The listing builds one solid part. Answer for the finished solid, in the listing's coordinates (mm). A direction names the side the tool comes from. Coordinates: 2 decimals unless noted, no trailing zeros. Write each loop counter-clockwise with the first axis right and the second up, starting at its lowest first coordinate (ties: lowest second). Pieces come first, ordered by that corner, then holes.
```python
from build123d import *

# Parameters (mm, degrees)
CROQUIS1_W              = 5.95
CROQUIS1_H              = 5.95
SALIENTE_EXTRUIR1_DEPTH = 3.5
CROQUIS3_R              = 1.7
SALIENTE_EXTRUIR2_DEPTH = 1.5
CROQUIS4_R              = 0.5
SALIENTE_EXTRUIR3_DEPTH = 0.4
CROQUIS5_W              = 1.355791782
CROQUIS5_H              = 0.82
SALIENTE_EXTRUIR4_DEPTH = 0.405
REDONDEO1_R             = 0.3
REDONDEO2_R             = 0.3
CROQUIS9_W              = 1.36
CROQUIS9_H              = 0.82
SALIENTE_EXTRUIR5_DEPTH = 0.405
REDONDEO3_R             = 0.3
REDONDEO4_R             = 0.3
CORTAR_EXTRUIR1_DEPTH   = 10.958472837


with BuildPart() as part:
    # Croquis1 → Saliente-Extruir1 (new body)
    with BuildSketch(Plane.XY):
        with Locations((-2.975, 2.975)):
            Rectangle(CROQUIS1_W, CROQUIS1_H)
    extrude(amount=SALIENTE_EXTRUIR1_DEPTH)

    # Croquis3 → Saliente-Extruir2 (add)
    with BuildSketch(Plane.XY.offset(3.5)):
        with Locations((-2.975, 2.975)):
            Circle(CROQUIS3_R)
    extrude(amount=SALIENTE_EXTRUIR2_DEPTH)

    # Croquis4 → Saliente-Extruir3 (add)
    with BuildSketch(Plane.XY.offset(3.5)):
        with Locations((-5.25, 5.3125)):
            Circle(CROQUIS4_R)
        with Locations(Location((-0.7, 5.3125, 0), (0, 0, 180))):
            Circle(CROQUIS4_R)
        with Locations((-0.7, 0.6375)):
            Circle(CROQUIS4_R)
        with Locations(Location((-5.25, 0.6375, 0), (0, 0, 180))):
            Circle(CROQUIS4_R)
    extrude(amount=SALIENTE_EXTRUIR3_DEPTH)

    # Croquis5 → Saliente-Extruir4 (add)
    with BuildSketch(Plane(origin=(0, 0, 0), x_dir=(0, 0, -1), z_dir=(1, 0, 0))):
        with Locations((-0.677895891, 5.4025)):
            Rectangle(CROQUIS5_W, CROQUIS5_H)
        with Locations((-0.677895891, 0.5475)):
            Rectangle(CROQUIS5_W, CROQUIS5_H)
    extrude(amount=SALIENTE_EXTRUIR4_DEPTH)

    # Redondeo1
    redondeo1_edges = [part.edges().sort_by_distance(p)[0] for p in [
        (0.405, 5.4025, 1.355791782),
    ]]
    fillet(redondeo1_edges, radius=REDONDEO1_R)

    # Redondeo2
    redondeo2_edges = [part.edges().sort_by_distance(p)[0] for p in [
        (0.405, 0.5475, 1.355791782),
    ]]
    fillet(redondeo2_edges, radius=REDONDEO2_R)

    # Croquis9 → Saliente-Extruir5 (add)
    with BuildSketch(Plane.ZY.offset(5.95)):
        with Locations((0.68, 5.4025)):
            Rectangle(CROQUIS9_W, CROQUIS9_H)
        with Locations((0.68, 0.5475)):
            Rectangle(CROQUIS9_W, CROQUIS9_H)
    extrude(amount=SALIENTE_EXTRUIR5_DEPTH)

    # Redondeo3
    redondeo3_edges = [part.edges().sort_by_distance(p)[0] for p in [
        (-6.355, 5.4025, 1.36),
    ]]
    fillet(redondeo3_edges, radius=REDONDEO3_R)

    # Redondeo4
    redondeo4_edges = [part.edges().sort_by_distance(p)[0] for p in [
        (-6.355, 0.5475, 1.36),
    ]]
    fillet(redondeo4_edges, radius=REDONDEO4_R)

    # Croquis10 → Cortar-Extruir1 (cut, through all)
    with BuildSketch(Plane.XZ.offset(-0.1375)):
        with BuildLine():
            Line((-5.95, 0), (-6.055, 0))
            Line((-6.055, 0), (-6.055, 0.955))
            ThreePointArc((-6.055, 0.955), (-6.024246212, 1.029246212), (-5.95, 1.06))
            Line((-5.95, 1.06), (-5.95, 0))
        make_face()
        with BuildLine():
            Line((0.105, 0), (0.105, 0.955))
            ThreePointArc((0.105, 0.955), (0.074246212, 1.029246212), (0, 1.06))
            Line((0, 1.06), (0, 0))
            Line((0, 0), (0.105, 0))
        make_face()
    extrude(amount=-CORTAR_EXTRUIR1_DEPTH, mode=Mode.SUBTRACT)


solid = part.part
```
(1) Section C-C, the plane y = 0.5 is taken. Write down the section's boundary in (x, z) (3 decimals), plus the area to 3 significant figures.
(2) Section D-D, the plane z = 2.35 is taken. Write down the section's boundary in (x, y).
(3) Which of the six approach directions +Z, -Z, +X, -X, +Y, -Y give full straight-line access (tool end or side, diameter ignored) to faces 1 (the flat face through (-4.34, 1.69, 3.5)), 2 (the flat face through (-0.7, 0.6, 3.9))?
(4) Each of these flat-tipped pins is pushed along its axis until it touches: pin 1 (1.8 mm diameter, centred on y = 2, z = 2, fed in from +X); pin 2 (1.1 mm diameter, centred on x = -0.5, y = 1, fed in from +Z). Where does it stop, or does it pass through?
(5) Section A-A, the plane z = 0.4 is taken. State how many separate pieces and enclosed holes the cut face has, plus the area to 3 significant figures.
(6) For a pull along X with two mould halves and no side action, classify faces 3 (the flat face through (0.405, 0.6, 0.5)), 4 (the flat face through (-0.7, 5.3, 3.9)), 5 (the cylindrical face through (-0.635, 4.817, 3.697)) as pulls with the +X half, pulls with the -X half, needs draft (parallel to the pull), parting line crosses it, or undercut.
(7) Section B-B, the plane x = -5.25 is taken. Write down the section's boundary in (y, z).
(8) Find the intervals of material crossed by probe 1 along Z at (x, y) = (-0.5, 0.3); probe 2 along X at (y, z) = (3.1, 1.3); probe 3 along Z at (x, y) = (-4.5, 4.2), in increasing order.
Solution:
1. outline: (-6.355, 0) - (-6.055, 0) - (-6.055, 0.955) arc R0.105 cw to (-5.95, 1.06) - (-5.95, 0) - (0, 0) - (0, 1.06) arc R0.105 cw to (0.105, 0.955) - (0.105, 0) - (0.405, 0) - (0.405, 1.056) arc R0.3 ccw to (0.105, 1.356) - (0, 1.356) - (0, 3.5) - (-0.219, 3.5) - (-0.219, 3.9) - (-1.181, 3.9) - (-1.181, 3.5) - (-4.769, 3.5) - (-4.769, 3.9) - (-5.731, 3.9) - (-5.731, 3.5) - (-5.95, 3.5) - (-5.95, 1.36) - (-6.055, 1.36) arc R0.3 ccw to (-6.355, 1.06) - close
1. area: 22.4 mm2
2. outline: (-5.95, 0) - (0, 0) - (0, 5.95) - (-5.95, 5.95) - close
3. face 1: +Z
3. face 2: +Z, +X, -X, +Y, -Y
4. pin 1: stops at x = 0
4. pin 2: stops at z = 3.9
5. separate pieces: 5
5. enclosed holes: 0
5. area: 36.4 mm2
6. face 3: pulls with the +X half
6. face 4: needs draft
6. face 5: undercut
7. outline: (0, 0) - (5.95, 0) - (5.95, 3.5) - (5.81, 3.5) - (5.81, 3.9) - (4.81, 3.9) - (4.81, 3.5) - (1.14, 3.5) - (1.14, 3.9) - (0.14, 3.9) - (0.14, 3.5) - (0, 3.5) - close
8. probe 1: z = 0 to 3.9
8. probe 2: x = -5.95 to 0
8. probe 3: z = 0 to 3.5
